Autodesk Inventor part; units mm, degrees
ref_plane "YZ Plane" through (0, 0, 0) normal (1, 0, 0) x (0, 1, 0)
ref_plane "XZ Plane" through (0, 0, 0) normal (0, 1, 0) x (-1, 0, 0)
ref_plane "XY Plane" through (0, 0, 0) normal (0, 0, 1) x (1, 0, 0)
sketch "Sketch1" plane through (0, 0, 0) normal (0, 0, 1) x (1, 0, 0)
  line L0 (-130.5517, -4.3675) -> (961.6483, -4.3675)
  line L1 (961.6483, -4.3675) -> (961.6483, 478.2325)
  line L2 (961.6483, 478.2325) -> (-130.5517, 478.2325)
  line L3 (-130.5517, 478.2325) -> (-130.5517, -4.3675)
  arc A0 (155.1983, 398.8575) -> (155.1983, 367.1075) centre (155.1983, 382.9825) ccw
  arc A1 (218.6983, 367.1075) -> (218.6983, 398.8575) centre (218.6983, 382.9825) ccw
  line L4 (155.1983, 398.8575) -> (218.6983, 398.8575)
  line L5 (218.6983, 367.1075) -> (155.1983, 367.1075)
  arc A2 (612.3983, 400.445) -> (612.3983, 368.695) centre (612.3983, 384.57) ccw
  arc A3 (675.8983, 368.695) -> (675.8983, 400.445) centre (675.8983, 384.57) ccw
  line L6 (612.3983, 400.445) -> (675.8983, 400.445)
  line L7 (675.8983, 368.695) -> (612.3983, 368.695)
  circle A4 centre (110.7483, 440.1325) radius 3.175
  circle A5 centre (110.7483, 414.7325) radius 3.175
  circle A6 centre (720.3483, 440.1325) radius 3.175
  circle A7 centre (720.3483, 414.7325) radius 3.175
  dimension "d0" = 1092.2
  dimension "d1" = 482.6
  dimension "d4" = 63.5
  dimension "d5" = 95.25
  dimension "d6" = 285.75
  dimension "d7" = 63.5
  dimension "d9" = 285.75
  dimension "d14" = 38.1
  dimension "d15" = 63.5
  dimension "d16" = 241.3
  dimension "d17" = 241.3
  dimension "d18" = 38.1
  dimension "d19" = 63.5
  dimension "d20" = 850.9
  dimension "d21" = 850.9
  dimension "d24" = 15.875
extrude "Extrusion1" add sketch "Sketch1" along normal blind 6.35
properties part number "FE-00011"
Geometry: final body of the model. Coordinates: model frame, mm. Round coordinates to 2 decimals unless told otherwise and drop trailing zeros. Loops run counter-clockwise (first coordinate to the right, second up) from the corner with the lowest first, then second, coordinate; pieces in that order, holes last.
Item 1: Contact query for flat-ended pins moving along their axis: P1, Ø7.5, axis at x = 720.35, y = 414.73, coming from the -Z side; P2, Ø4, axis at x = 110.75, y = 440.13, coming from the +Z side. Output: stop coordinate, or through.
Checked values:
P1: stops at z = 0
P2: passes through
Item 2: Mould query, pull axis Z, two halves, no side actions, for faces 1 (the flat face through (408, 240, 6.35)), 2 (the flat face through (408, 240, 0)). Classes: released by +Z, released by -Z, zero draft, split by the parting line, or undercut.
Checked values:
face 1: released by +Z
face 2: released by -Z
Item 3: Line query: L1, parallel to X at y = 439.5, z = 1.25; L2, parallel to X at y = 443, z = 3.75. Output: solid intervals per line, ascending.
Checked values:
L1: x = -130.55 to 107.64, 113.86 to 717.24, 723.46 to 961.65
L2: x = -130.55 to 109.39, 112.11 to 718.99, 721.71 to 961.65
Item 4: Section A-A, the plane y = 384.57. Output: boundary loops of the cut face in (x, z).
Checked values:
outline: (-130.55, 0) - (139.4, 0) - (139.4, 6.35) - (-130.55, 6.35) - close; (234.49, 0) - (596.52, 0) - (596.52, 6.35) - (234.49, 6.35) - close; (691.77, 0) - (961.65, 0) - (961.65, 6.35) - (691.77, 6.35) - close
